from build123d import *

# Parameters (mm, degrees)
SKETCH1_W           = 4.7
SKETCH1_H           = 11.8
SKETCH1_R           = 1
BOSS_EXTRUDE1_DEPTH = 2
SKETCH2_W           = 4.7
SKETCH2_H           = 1
BOSS_EXTRUDE2_DEPTH = 8
SKETCH3_R           = 1.5
CUT_EXTRUDE1_DEPTH  = 8


with BuildPart() as part:
    # Sketch1 → Boss-Extrude1 (new body)
    with BuildSketch(Plane.XY):
        with Locations((2.35, 5.9)):
            Rectangle(SKETCH1_W, SKETCH1_H)
        with Locations((2.35, 5.9)):
            Circle(SKETCH1_R, mode=Mode.SUBTRACT)
    extrude(amount=BOSS_EXTRUDE1_DEPTH)

    # Sketch2 → Boss-Extrude2 (add)
    with BuildSketch(Plane(origin=(0, 0, 0), x_dir=(-1, 0, 0), z_dir=(0, 0, -1))):
        with Locations((-2.35, 0.5)):
            Rectangle(SKETCH2_W, SKETCH2_H)
    extrude(amount=BOSS_EXTRUDE2_DEPTH)

    # Sketch3 → Cut-Extrude1 (cut)
    with BuildSketch(Plane(origin=(0, 1, 0), x_dir=(1, 0, 0), z_dir=(0, 1, 0))):
        with Locations((2.35, 2)):
            Circle(SKETCH3_R)
        with Locations((2.35, 6)):
            Circle(SKETCH3_R)
    extrude(amount=-CUT_EXTRUDE1_DEPTH, mode=Mode.SUBTRACT)


solid = part.part
The model under review builds one solid part; all positions refer to its coordinate system, in mm. A direction names the side the tool comes from. Round coordinates to 2 decimals unless told otherwise and drop trailing zeros. Write each loop counter-clockwise with the first axis right and the second up, starting at its lowest first coordinate (ties: lowest second). Pieces come first, ordered by that corner, then holes. Notation, with made-up numbers: (22, 33.25) - (56, 33.25) arc R23 cw to (56, 48.25) - close; hole circle Ø10 at (-19, 39.5). An arc over 180 degrees is marked (long way). One line per item, written item: value. Start each with the question number.
1. Consider section D-D on x = 0.4. Write out the cut boundary in (y, z), and give its area (3 significant figures).
2. The part is to be moulded in two halves that separate along X. For faces 1 (the face through (0, 4.6, 0.4)), 2 (the face through (2.81, 5.01, 0.99)), 3 (the face through (1, 6, 2)), say which applies: released by +X, released by -X, zero draft, split by the parting line, or undercut.
3. Consider section C-C on z = 1.5. Write out the cut boundary in (x, y).
4. Consider section B-B on y = 6.5. Write out the cut boundary in (x, z), and give its area (3 significant figures).
5. Clearance check with a flat-ended pin moving along its axis: P1, Ø2.5, axis at x = 3.5, z = -2.5, coming from the +Y side. State where the tip first meets the part, or that it passes through.
6. Consider section A-A on z = -2. Write out the cut boundary in (x, y), and give its area (3 significant figures).
7. Machinability: for faces 4 (the face through (2, 1, -4)), 5 (the face through (2.4, 0.5, -8)), which of the approach directions +Z, -Z, +X, -X, +Y, -Y give a long, thin tool a straight path to every point of the face, cutting with its end or side? Answer none if there is none.
8. To check wall thickness, follow L1, parallel to Z at x = 2.35, y = 0.8; L2, parallel to X at y = 0.5, z = -6; L3, parallel to Z at x = 1.85, y = 10.75. State the ranges of each line that lie inside material, in increasing order. Write a range as from..to.
Checks:
1. outline: (0, -8) - (1, -8) - (1, 0) - (11.8, 0) - (11.8, 2) - (0, 2) - close
1. area: 31.6 mm^2
2. face 1: released by -X
2. face 2: undercut
2. face 3: zero draft
3. outline: (0, 0) - (4.7, 0) - (4.7, 11.8) - (0, 11.8) - close; hole circle Ø2 at (2.35, 5.9)
4. outline: (0, 0) - (1.55, 0) - (1.55, 2) - (0, 2) - close; (3.15, 0) - (4.7, 0) - (4.7, 2) - (3.15, 2) - close
4. area: 6.20 mm^2
5. P1: stops at y = 1
6. outline: (0, 0) - (0.85, 0) - (0.85, 1) - (0, 1) - close; (3.85, 0) - (4.7, 0) - (4.7, 1) - (3.85, 1) - close
6. area: 1.70 mm^2
7. face 4: -Z, +X, -X, +Y
7. face 5: -Z, +X, -X, +Y, -Y
8. L1: z = -8..-7.5, -4.5..-3.5, -0.5..2
8. L2: x = 0..0.85, 3.85..4.7
8. L3: z = 0..2
